Source: CAD feature listing. Evaluate the final solid. Frame: model axes, mm. A direction names the side the tool comes from. Coordinates: 2 decimals unless noted, no trailing zeros. Order: outer loops, then holes, each group sorted by start corner. A loop starts at its lowest first (then second) coordinate and runs counter-clockwise, first axis right, second up.
```python
from build123d import *

# Parameters (mm, degrees)
BOSS_EXTRUDE1_DEPTH = 12
SKETCH2_R           = 1.5
BOSS_EXTRUDE2_DEPTH = 8
SKETCH3_R           = 1.5
CUT_EXTRUDE1_DEPTH  = 8
CHAMFER1_SIZE       = 0.3


with BuildPart() as part:
    # Sketch1 → Boss-Extrude1 (new body)
    with BuildSketch(Plane(origin=(0, 0, 0), x_dir=(0, 0, -1), z_dir=(1, 0, 0))):
        Polygon((0, 3.175426481), (-2.75, 1.58771324), (-2.75, -1.58771324), (0, -3.175426481), (2.75, -1.58771324), (2.75, 1.58771324), align=None)
    extrude(amount=BOSS_EXTRUDE1_DEPTH)

    # Sketch2 → Boss-Extrude2 (add)
    with BuildSketch(Plane(origin=(12, 0, 0), x_dir=(0, 0, -1), z_dir=(1, 0, 0))):
        Circle(SKETCH2_R)
    extrude(amount=BOSS_EXTRUDE2_DEPTH)

    # Sketch3 → Cut-Extrude1 (cut)
    with BuildSketch(Plane.ZY):
        with Locations(Location((0, 0, 0), (0, 0, 180))):
            Circle(SKETCH3_R)
    extrude(amount=-CUT_EXTRUDE1_DEPTH, mode=Mode.SUBTRACT)

    # Sketch4 → Cut-Revolve1 (revolve, cut)
    with BuildSketch(Plane(origin=(0, 0, 0), x_dir=(1, 0, 0), z_dir=(0, 1, 0)), mode=Mode.PRIVATE) as cut_revolve1_sk:
        Polygon((0, 10.219809024), (4.392081913, 10.219809024), (0, 2.6125), align=None)
        Polygon((12, 2.6125), (12, 10.219809024), (7.607918087, 10.219809024), align=None)
    revolve(cut_revolve1_sk.sketch.rotate(Axis((0, 0, 0), (-1, 0, 0)), 210.000000006), axis=Axis((0, 0, 0), (-1, 0, 0)), mode=Mode.SUBTRACT)

    # Chamfer1
    chamfer1_edges = [part.edges().sort_by_distance(p)[0] for p in [
        (20, 0, 1.5),
    ]]
    chamfer(chamfer1_edges, length=CHAMFER1_SIZE)


solid = part.part
```
1. Section query C-C, the plane x = 10.75. Output: boundary loops of the cut face in (y, z), plus the area to 3 significant figures.
2. Material intervals for line 1 along X through (y, z) = (2, -1.15); line 2 along X through (y, z) = (0.5, 0.4); line 3 along Y through (x, z) = (17, -0.9), sorted ascending.
3. Section query B-B, the plane y = 0. Output: boundary loops of the cut face in (x, z).
4. Draft query along Y for faces 4 (the flat face through (6, 0, -2.75)), 5 (the cylindrical face through (15.8, 0.07, 1.5)), 6 (the flat face through (8, 0, 0)). Return one class per face: +Y half, -Y half, draft (parallel to the pull), parting line (faces both ways), or undercut.
5. Access query for faces 1 (the cylindrical face through (3.94, -0.45, -1.43)), 2 (the flat face through (12, -2, 0)), 3 (the flat face through (5.92, -2.39, -1.36)). Directions: +Z, -Z, +X, -X, +Y, -Y. A direction counts if a zero-diameter tool reaches every point of the face in a straight line with its end or side. Return the directions, or none.
6. Contact query for flat-ended pins moving along their axis: P1, Ø1.5, axis at x = 3, z = 2, coming from the +Y side; P2, Ø1.5, axis at y = 0, z = 0.5, coming from the -X side; P3, Ø2, axis at x = 18, z = 1.5, coming from the +Y side. Output: stop coordinate, or through.
7. Section query A-A, the plane x = 6.5. Output: boundary loops of the cut face in (y, z).
Answer key:
1. outline: (-3.18, 0) - (-1.59, -2.75) - (1.59, -2.75) - (3.18, 0) - (1.59, 2.75) - (-1.59, 2.75) - close
1. area: 26.2 mm2
2. line 1: x = 0 to 12
2. line 2: x = 8 to 20
2. line 3: y = -1.2 to 1.2
3. outline: (0, -2.61) - (0.08, -2.75) - (11.92, -2.75) - (12, -2.61) - (12, -1.5) - (19.7, -1.5) - (20, -1.2) - (20, 1.2) - (19.7, 1.5) - (12, 1.5) - (12, 2.61) - (11.92, 2.75) - (0.08, 2.75) - (0, 2.61) - (0, 1.5) - (8, 1.5) - (8, -1.5) - (0, -1.5) - close
4. face 4: draft
4. face 5: parting line
4. face 6: undercut
5. face 1: -X
5. face 2: +X
5. face 3: -Z, +X, -X, -Y
6. P1: stops at y = 2.45
6. P2: stops at x = 8
6. P3: stops at y = 1.41
7. outline: (-3.18, 0) - (-1.59, -2.75) - (1.59, -2.75) - (3.18, 0) - (1.59, 2.75) - (-1.59, 2.75) - close; hole circle Ø3 at (0, 0)
